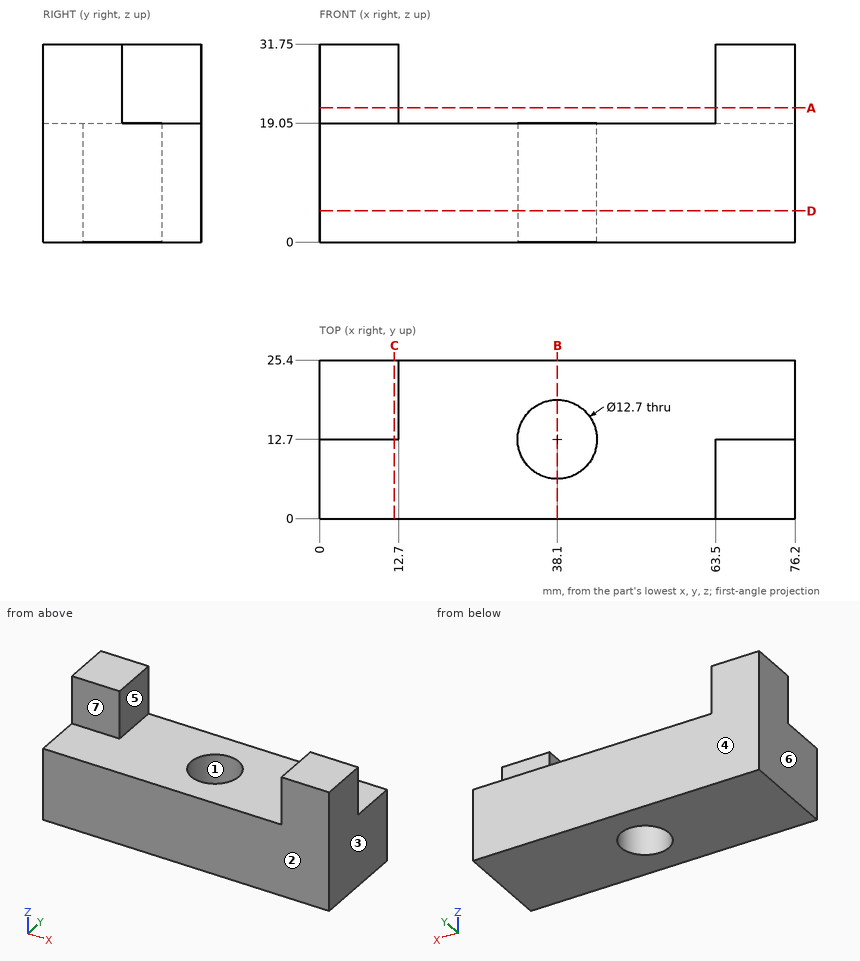
Here's the drawing with two shaded views (mm, measured from the low corner). I have some questions. A direction names the side the tool comes from. Coordinates: 2 decimals unless noted, no trailing zeros. Write each loop counter-clockwise with the first axis right and the second up, starting at its lowest first coordinate (ties: lowest second). Pieces come first, ordered by that corner, then holes.
Item 1: On a 3-axis mill with a long thin cutter (end or side, diameter ignored), from which of +Z, -Z, +X, -X, +Y, -Y can I reach the whole of each face in a straight line? I mean the marked faces 5, 6 and 7. Say none if no direction works.
Item 2: I want a section at A-A on z = 21.5. Write out the boundary of the cut face in (x, y), and give its area (3 significant figures).
Item 3: If we mould it in two halves opening along Y, with no side actions, what happens to the marked faces 1, 2, 3 and 4? For each: +Y half, -Y half, draft (parallel to the pull), parting line (faces both ways), or undercut.
Item 4: If I drill on line 1 (Y direction, x = 38.1, z = 12.5); line 2 (Z direction, x = 26, y = 23.5); line 3 (X direction, y = 12.7, z = 4.75), over which ranges is the centre line in solid material (lowest first)?
Item 5: Will these pins go through, and if not, where does the flat tip stop? pin 1 (2 mm diameter, centred on y = 22.5, z = 20.5, fed in from +X); pin 2 (10 mm diameter, centred on y = 3.5, z = 24.5, fed in from -X); pin 3 (11.5 mm diameter, centred on x = 38.1, y = 12.7, fed in from +Z); pin 4 (6 mm diameter, centred on x = 12, z = 24.5, fed in from -Y).
Item 6: I want a section at B-B on x = 38.1. Write out the boundary of the cut face in (y, z).
Item 7: I want a section at C-C on x = 12. Write out the boundary of the cut face in (y, z).
Item 8: I want a section at D-D on z = 5. Write out the boundary of the cut face in (x, y), and give its area (3 significant figures).
Findings below:
1. face 5: +Z, +X, +Y, -Y
1. face 6: +Z, -Z, -X, +Y, -Y
1. face 7: +Z, -X, -Y
2. outline: (0, 12.7) - (12.7, 12.7) - (12.7, 25.4) - (0, 25.4) - close; (63.5, 0) - (76.2, 0) - (76.2, 12.7) - (63.5, 12.7) - close
2. area: 323 mm2
3. face 1: undercut
3. face 2: -Y half
3. face 3: draft
3. face 4: +Y half
4. line 1: y = 0 to 6.35, 19.05 to 25.4
4. line 2: z = 0 to 19.05
4. line 3: x = 0 to 31.75, 44.45 to 76.2
5. pin 1: stops at x = 12.7
5. pin 2: stops at x = 63.5
5. pin 3: passes through
5. pin 4: stops at y = 12.7
6. outline: (0, 0) - (6.35, 0) - (6.35, 19.05) - (0, 19.05) - close; (19.05, 0) - (25.4, 0) - (25.4, 19.05) - (19.05, 19.05) - close
7. outline: (0, 0) - (25.4, 0) - (25.4, 31.75) - (12.7, 31.75) - (12.7, 19.05) - (0, 19.05) - close
8. outline: (0, 0) - (76.2, 0) - (76.2, 25.4) - (0, 25.4) - close; hole circle Ø12.7 at (38.1, 12.7)
8. area: 1,810 mm2
